Check sheet for the modelled part. Datum: model origin and axes. Units: mm. A direction names the side the tool comes from. Coordinates: 2 decimals unless noted, no trailing zeros. Loops run counter-clockwise (first coordinate to the right, second up) from the corner with the lowest first, then second, coordinate; pieces in that order, holes last. Notation, with made-up numbers: (78, 72) -> (107, 72) arc R24 cw to (107, 95) -> close; hole circle Ø6 at (73.5, 88.5). An arc over 180 degrees is marked (long way). Use one line per item in the form item = value.
from build123d import *

# Parameters (mm, degrees)
ESQUISSE1_W             = 199.383138687
ESQUISSE1_H             = 82.793301959
BOSS_EXTRU_1_DEPTH      = 10
ESQUISSE2_W             = 9.546755773
ESQUISSE2_H             = 82.793301959
BOSS_EXTRU_3_DEPTH      = 10
ESQUISSE3_W             = 7.522297827
ESQUISSE3_H             = 80.237843489
ENL_V_MAT_EXTRU_1_DEPTH = 6
ESQUISSE4_W             = 194.871216777
ESQUISSE4_H             = 77.918512405
ENL_V_MAT_EXTRU_2_DEPTH = 6
ESQUISSE5_W             = 5.655894549
ESQUISSE5_H             = 62.197790312
ENL_V_MAT_EXTRU_3_DEPTH = 6
CONG_1_R                = 2
CONG_2_R                = 2
CONG_3_R                = 2
CONG_4_R                = 2


with BuildPart() as part:
    # Esquisse1 → Boss.-Extru.1 (new body)
    with BuildSketch(Plane.XY):
        with Locations((99.691569344, 41.39665098)):
            Rectangle(ESQUISSE1_W, ESQUISSE1_H)
    extrude(amount=BOSS_EXTRU_1_DEPTH)

    # Esquisse2 → Boss.-Extru.3 (add)
    with BuildSketch(Plane(origin=(0, 0, 0), x_dir=(-1, 0, 0), z_dir=(0, 0, -1))):
        with Locations((-194.6097608, 41.39665098)):
            Rectangle(ESQUISSE2_W, ESQUISSE2_H)
    extrude(amount=BOSS_EXTRU_3_DEPTH)

    # Esquisse3 → Enlèv. mat.-Extru.1 (cut)
    with BuildSketch(Plane.ZY.offset(-189.836382914)):
        with Locations((-3.761148914, 41.217548651)):
            Rectangle(ESQUISSE3_W, ESQUISSE3_H)
    extrude(amount=-ENL_V_MAT_EXTRU_1_DEPTH, mode=Mode.SUBTRACT)

    # Esquisse4 → Enlèv. mat.-Extru.2 (cut)
    with BuildSketch(Plane(origin=(0, 0, 0), x_dir=(-1, 0, 0), z_dir=(0, 0, -1))):
        with Locations((-100.115772064, 42.377214193)):
            Rectangle(ESQUISSE4_W, ESQUISSE4_H)
    extrude(amount=-ENL_V_MAT_EXTRU_2_DEPTH, mode=Mode.SUBTRACT)

    # Esquisse5 → Enlèv. mat.-Extru.3 (cut)
    with BuildSketch(Plane(origin=(199.383138687, 0, 0), x_dir=(0, 0, -1), z_dir=(1, 0, 0))):
        with Locations((-2.827947275, 41.363585287)):
            Rectangle(ESQUISSE5_W, ESQUISSE5_H)
    extrude(amount=-ENL_V_MAT_EXTRU_3_DEPTH, mode=Mode.SUBTRACT)

    # Congé1
    cong_1_edges = [part.edges().sort_by_distance(p)[0] for p in [
        (199.383138687, 0, 0),
    ]]
    fillet(cong_1_edges, radius=CONG_1_R)

    # Congé2
    cong_2_edges = [part.edges().sort_by_distance(p)[0] for p in [
        (199.383138687, 82.793301959, 0),
    ]]
    fillet(cong_2_edges, radius=CONG_2_R)

    # Congé3
    cong_3_edges = [part.edges().sort_by_distance(p)[0] for p in [
        (0, 82.793301959, 5),
    ]]
    fillet(cong_3_edges, radius=CONG_3_R)

    # Congé4
    cong_4_edges = [part.edges().sort_by_distance(p)[0] for p in [
        (0, 0, 5),
    ]]
    fillet(cong_4_edges, radius=CONG_4_R)


solid = part.part
(1) Scan lines: line 1 along Y through (x, z) = (26, 2); line 2 along X through (y, z) = (77.5, 5.5); line 3 along Z through (x, y) = (146, 51). Record each from-to range of solid material in increasing order.
Established:
line_1 = 0 to 3.42, 81.34 to 82.79
line_2 = 0 to 2.68, 197.55 to 199.38
line_3 = 6 to 10
(2) Tool access check on faces 4 (the flat face through (193, 41, -7.522)), 5 (the flat face through (189.836, 41, -8)), 6 (the flat face through (98, 42, 10)). Record the directions out of +Z, -Z, +X, -X, +Y, -Y that give a thin tool (end or side, any length) a straight path to the whole face; none if there is none.
Established:
face_4 = -X
face_5 = -Z, -X, +Y, -Y
face_6 = +Z, +X, -X, +Y, -Y
(3) Section check A-A, the plane x = 155.5. Record the boundary of the cut face in (y, z).
Established:
outline = (0, 0) -> (3.42, 0) -> (3.42, 6) -> (81.34, 6) -> (81.34, 0) -> (82.79, 0) -> (82.79, 10) -> (0, 10) -> close
(4) Section check C-C, the plane z = 1.75. Record the boundary of the cut face in (x, y), plus the area to 3 significant figures.
Established:
outline = (0, 2) arc R2 ccw to (2, 0) -> (197.38, 0) arc R2 ccw to (199.38, 2) -> (199.38, 10.26) -> (197.55, 10.26) -> (197.55, 3.42) -> (2.68, 3.42) -> (2.68, 81.34) -> (197.55, 81.34) -> (197.55, 72.46) -> (199.38, 72.46) -> (199.38, 80.79) arc R2 ccw to (197.38, 82.79) -> (2, 82.79) arc R2 ccw to (0, 80.79) -> close
area = 1,210 mm²
(5) Mould release check, pull along Z, two halves, no side actions. Record for faces 1 (the flat face through (2.68, 42, 3)), 2 (the flat face through (195, 42, -10)), 3 (the flat face through (193, 1.099, -4)): +Z half, -Z half, draft (parallel to the pull), parting line (faces both ways), or undercut.
Established:
face_1 = draft
face_2 = -Z half
face_3 = undercut
(6) Section check D-D, the plane y = 77.5. Record the boundary of the cut face in (x, z), plus the area to 3 significant figures.
Established:
outline = (0, 0) -> (2.68, 0) -> (2.68, 6) -> (197.55, 6) -> (197.55, 0) -> (195.84, 0) -> (195.84, -7.52) -> (189.84, -7.52) -> (189.84, -10) -> (199.38, -10) -> (199.38, 10) -> (0, 10) -> close
area = 875 mm²
(7) Section check B-B, the plane y = 53. Record the boundary of the cut face in (x, z).
Established:
outline = (0, 0) -> (2.68, 0) -> (2.68, 6) -> (197.55, 6) -> (197.55, 5.66) -> (199.38, 5.66) -> (199.38, 10) -> (0, 10) -> close; (189.84, -10) -> (199.38, -10) -> (199.38, 0) -> (195.84, 0) -> (195.84, -7.52) -> (189.84, -7.52) -> close
(8) Go/stop test with flat-tipped pins: P1, Ø0.9, axis at x = 198.5, z = 1.5, coming from the -Y side; P2, Ø1.5, axis at x = 198.5, z = 4, coming from the +Y side; P3, Ø3, axis at y = 42, z = 4, coming from the +X side; P4, Ø10, axis at x = 163, z = -6.5, coming from the -Y side. Record where each tip stops, or that it passes through.
Established:
P1 = 0.11
P2 = 82.76
P3 = 2.68
P4 = through
